Can you work these out from the model? Positions are in its coordinate system, mm. A direction names the side the tool comes from. Coordinates: 2 decimals unless noted, no trailing zeros. Order: outer loops, then holes, each group sorted by start corner. A loop starts at its lowest first (then second) coordinate and runs counter-clockwise, first axis right, second up. Notation, with made-up numbers: (79, -37) -> (129, -37) arc R13 cw to (129, -32) -> close; hole circle Ø2 at (-13, 7.25). An arc over 180 degrees is marked (long way). Answer in a Markdown table with one row per item. Add a question column.
1. On a 3-axis mill with a long thin cutter (end or side, diameter ignored), from which of +Z, -Z, +X, -X, +Y, -Y can I reach the whole of each face in a straight line? I mean faces 1 (the face through (-0.59, 4.46, 34.52)), 2 (the face through (-5.8, -14, 18)), 3 (the face through (-1, -4.51, 14.12)). Say none if no direction works.
2. We'd pull the mould along Z, two halves only. Please class faces 4 (the face through (0, -6, 37)), 5 (the face through (0, 10, 18)), 6 (the face through (4, -4, 30)): pulls with the +Z half, pulls with the -Z half, needs draft (parallel to the pull), parting line crosses it, or undercut.
3. If I drill on line 1 along X through (y, z) = (0, 18.7) (3 decimals); line 2 along Y through (x, z) = (0, 25.3) (3 decimals); line 3 along Z through (x, y) = (1, 7.75), over which ranges is the centre line in solid material (lowest first)? Write a range as [from, to].
4. Imagine slicing it at A-A on z = 18.5. Write out the boundary of the cut face in (x, y) (3 decimals).
5. Imagine slicing it at B-B on x = -7.25. State how many separate pieces and enclosed holes the cut face has, plus the area to 3 significant figures.
from build123d import *

# Parameters (mm, degrees)
CROQUIS1_R              = 10
CROQUIS1_R_2            = 4.365
SALIENTE_EXTRUIR1_DEPTH = 37
CORTAR_EXTRUIR1_START   = 1
CROQUIS1_3_R            = 8.5
CORTAR_EXTRUIR1_DEPTH   = 5
CORTAR_EXTRUIR2_START   = 7
CROQUIS1_4_R            = 8.5
CORTAR_EXTRUIR2_DEPTH   = 5
CORTAR_EXTRUIR3_START   = 13
CROQUIS1_5_R            = 8.5
CORTAR_EXTRUIR3_DEPTH   = 5
CORTAR_EXTRUIR4_START   = 19
CROQUIS1_6_R            = 8.5
CORTAR_EXTRUIR4_DEPTH   = 5
CORTAR_EXTRUIR5_START   = 25
CROQUIS1_7_R            = 8.5
CORTAR_EXTRUIR5_DEPTH   = 5
CHAFL_N1_SIZE           = 5
CORTAR_EXTRUIR6_START   = 37
CROQUIS4_R              = 4.5
CORTAR_EXTRUIR6_DEPTH   = 4
CHAFL_N2_SIZE           = 1
SALIENTE_EXTRUIR2_DEPTH = 37
CORTAR_EXTRUIR7_START   = -10
CROQUIS6_R              = 3.3
CORTAR_EXTRUIR7_DEPTH   = 116
CORTAR_EXTRUIR8_START   = -12
CORTAR_EXTRUIR8_DEPTH   = 5


with BuildPart() as part:
    # Croquis1 → Saliente-Extruir1 (new body)
    with BuildSketch(Plane.XY):
        Circle(CROQUIS1_R)
        Circle(CROQUIS1_R_2, mode=Mode.SUBTRACT)
    extrude(amount=SALIENTE_EXTRUIR1_DEPTH)

    # Croquis1<3> → Cortar-Extruir1 (cut)
    with BuildSketch(Plane.XY.offset(CORTAR_EXTRUIR1_START)):
        Circle(CROQUIS1_3_R)
    extrude(amount=CORTAR_EXTRUIR1_DEPTH, mode=Mode.SUBTRACT)

    # Croquis1<4> → Cortar-Extruir2 (cut)
    with BuildSketch(Plane.XY.offset(CORTAR_EXTRUIR2_START)):
        Circle(CROQUIS1_4_R)
    extrude(amount=CORTAR_EXTRUIR2_DEPTH, mode=Mode.SUBTRACT)

    # Croquis1<5> → Cortar-Extruir3 (cut)
    with BuildSketch(Plane.XY.offset(CORTAR_EXTRUIR3_START)):
        Circle(CROQUIS1_5_R)
    extrude(amount=CORTAR_EXTRUIR3_DEPTH, mode=Mode.SUBTRACT)

    # Croquis1<6> → Cortar-Extruir4 (cut)
    with BuildSketch(Plane.XY.offset(CORTAR_EXTRUIR4_START)):
        Circle(CROQUIS1_6_R)
    extrude(amount=CORTAR_EXTRUIR4_DEPTH, mode=Mode.SUBTRACT)

    # Croquis1<7> → Cortar-Extruir5 (cut)
    with BuildSketch(Plane.XY.offset(CORTAR_EXTRUIR5_START)):
        Circle(CROQUIS1_7_R)
    extrude(amount=CORTAR_EXTRUIR5_DEPTH, mode=Mode.SUBTRACT)

    # Chaflán1
    # the kernel refuses this chamfer: 5 mm, written as the material it adds along each edge
    with BuildSketch(Plane(origin=(0, 0, 13), x_dir=(1, 0, 0), z_dir=(0, -1, 0))) as chafl_n1_piece_1_section:
        Polygon((8.5 - CHAFL_N1_SIZE, 0), (8.5, CHAFL_N1_SIZE), (8.5, 0), align=None)
    chafl_n1_piece_1 = revolve(axis=Axis((0, 0, 13), (0, 0, 1)), mode=Mode.PRIVATE)
    chafl_n1_piece_1 = chafl_n1_piece_1 - Plane(origin=(0, 0, 15.944314862), x_dir=(1, 0, 0), z_dir=(0, 0, -1)) * Cylinder(4.365, 34, mode=Mode.PRIVATE)
    add(chafl_n1_piece_1)
    with BuildSketch(Plane(origin=(0, 0, 7), x_dir=(1, 0, 0), z_dir=(0, -1, 0))) as chafl_n1_piece_2_section:
        Polygon((8.5 - CHAFL_N1_SIZE, 0), (8.5, CHAFL_N1_SIZE), (8.5, 0), align=None)
    chafl_n1_piece_2 = revolve(axis=Axis((0, 0, 7), (0, 0, 1)), mode=Mode.PRIVATE)
    chafl_n1_piece_2 = chafl_n1_piece_2 - Plane(origin=(0, 0, 9.944314862), x_dir=(1, 0, 0), z_dir=(0, 0, -1)) * Cylinder(4.365, 34, mode=Mode.PRIVATE)
    add(chafl_n1_piece_2)
    with BuildSketch(Plane(origin=(0, 0, 1), x_dir=(1, 0, 0), z_dir=(0, -1, 0))) as chafl_n1_piece_3_section:
        Polygon((8.5 - CHAFL_N1_SIZE, 0), (8.5, CHAFL_N1_SIZE), (8.5, 0), align=None)
    chafl_n1_piece_3 = revolve(axis=Axis((0, 0, 1), (0, 0, 1)), mode=Mode.PRIVATE)
    chafl_n1_piece_3 = chafl_n1_piece_3 - Plane(origin=(0, 0, 3.944314862), x_dir=(1, 0, 0), z_dir=(0, 0, -1)) * Cylinder(4.365, 34, mode=Mode.PRIVATE)
    add(chafl_n1_piece_3)
    with BuildSketch(Plane(origin=(0, 0, 25), x_dir=(1, 0, 0), z_dir=(0, -1, 0))) as chafl_n1_piece_4_section:
        Polygon((8.5, CHAFL_N1_SIZE), (8.5 - CHAFL_N1_SIZE, 0), (8.5, 0), align=None)
    chafl_n1_piece_4 = revolve(axis=Axis((0, 0, 25), (0, 0, 1)), mode=Mode.PRIVATE)
    chafl_n1_piece_4 = chafl_n1_piece_4 - Plane(origin=(0, 0, 27.944314862), x_dir=(1, 0, 0), z_dir=(0, 0, -1)) * Cylinder(4.365, 34, mode=Mode.PRIVATE)
    add(chafl_n1_piece_4)
    with BuildSketch(Plane(origin=(0, 0, 19), x_dir=(1, 0, 0), z_dir=(0, -1, 0))) as chafl_n1_piece_5_section:
        Polygon((8.5, CHAFL_N1_SIZE), (8.5 - CHAFL_N1_SIZE, 0), (8.5, 0), align=None)
    chafl_n1_piece_5 = revolve(axis=Axis((0, 0, 19), (0, 0, 1)), mode=Mode.PRIVATE)
    chafl_n1_piece_5 = chafl_n1_piece_5 - Plane(origin=(0, 0, 21.944314862), x_dir=(1, 0, 0), z_dir=(0, 0, -1)) * Cylinder(4.365, 34, mode=Mode.PRIVATE)
    add(chafl_n1_piece_5)

    # Croquis4 → Cortar-Extruir6 (cut)
    with BuildSketch(Plane.XY.offset(CORTAR_EXTRUIR6_START)):
        Circle(CROQUIS4_R)
    extrude(amount=-CORTAR_EXTRUIR6_DEPTH, mode=Mode.SUBTRACT)

    # Chaflán2
    chafl_n2_edges = [part.edges().sort_by_distance(p)[0] for p in [
        (-4.5, 0, 37),
    ]]
    chamfer(chafl_n2_edges, length=CHAFL_N2_SIZE)

    # Croquis5 → Saliente-Extruir2 (add)
    with BuildSketch(Plane.XY):
        with BuildLine():
            Line((10, -16.611303619), (10, 0))
            ThreePointArc((10, 0), (0, -10), (-10, 0))
            Line((-10, 0), (-10, -16.611303619))
            Line((-10, -16.611303619), (10, -16.611303619))
        make_face()
    extrude(amount=SALIENTE_EXTRUIR2_DEPTH)

    # Croquis6 → Cortar-Extruir7 (cut)
    with BuildSketch(Plane(origin=(0, 0, 0), x_dir=(1, 0, 0), z_dir=(0, 1, 0)).offset(CORTAR_EXTRUIR7_START)):
        with Locations(Location((0, -18.5, 0), (0, 0, 270))):
            Circle(CROQUIS6_R)
    extrude(amount=-CORTAR_EXTRUIR7_DEPTH, mode=Mode.SUBTRACT)

    # Croquis6<3> → Cortar-Extruir8 (cut)
    with BuildSketch(Plane(origin=(0, 0, 0), x_dir=(1, 0, 0), z_dir=(0, 1, 0)).offset(CORTAR_EXTRUIR8_START)):
        Polygon((0, -25.197263123), (5.8, -21.848631561), (5.8, -15.151368439), (0, -11.802736877), (-5.8, -15.151368439), (-5.8, -21.848631561), align=None)
    extrude(amount=-CORTAR_EXTRUIR8_DEPTH, mode=Mode.SUBTRACT)


solid = part.part
Answers follow:
| question | item | result |
|---|---|---|
| 1 | face 1 | +Z |
| 1 | face 2 | -Y |
| 1 | face 3 | none |
| 2 | face 4 | pulls with the +Z half |
| 2 | face 5 | needs draft |
| 2 | face 6 | undercut |
| 3 | line 1 | x = [-10, -4.365], [4.365, 10] |
| 3 | line 2 | y = [-16.611, -4.365], [4.365, 10] |
| 3 | line 3 | z = [0, 5.31], [6, 11.31], [12, 17.31], [18, 23.31], [24, 29.31], [30, 37] |
| 4 | outline | (-10, -16.611) -> (-5.8, -16.611) -> (-5.8, -12) -> (-3.3, -12) -> (-3.3, -10) -> (3.3, -10) -> (3.3, -12) -> (5.8, -12) -> (5.8, -16.611) -> (10, -16.611) -> (10, 0) arc R10 ccw to (-10, 0) -> close; hole circle Ø8.73 at (0, 0) |
| 5 | separate pieces | 1 |
| 5 | enclosed holes | 5 |
| 5 | area | 833 mm² |
